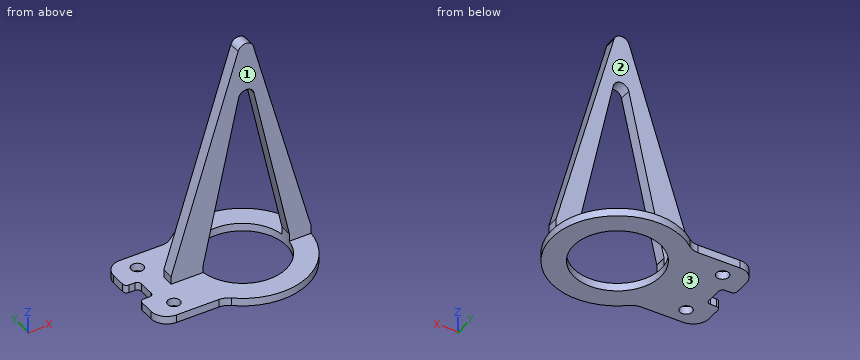
```python
from build123d import *

# Parameters (mm, degrees)
SKETCH_1_R          = 1.56
SKETCH_1_R_2        = 10.981035736
EXTRUDE_1_DEPTH     = 2
EXTRUDE_3_DEPTH     = 2
EXTRUDE_4_DEPTH     = 3
SKETCH_4_W          = 3.5
SKETCH_4_H          = 6
CUT_EXTRUDE_1_DEPTH = 10
FILLET_1_R          = 1
FILLET_2_R          = 1


with BuildPart() as part:
    # 草图1 → 凸台-拉伸1 (new body)
    with BuildSketch(Plane.XY):
        with BuildLine():
            Line((-13.173260362, 11.66726189), (-23.87331228, 11.66726189))
            ThreePointArc((-23.87331228, 11.66726189), (-26.701739405, 10.495689014), (-27.87331228, 7.66726189))
            Line((-27.87331228, 7.66726189), (-27.87331228, -7.66726189))
            ThreePointArc((-27.87331228, -7.66726189), (-26.701739405, -10.495689014), (-23.87331228, -11.66726189))
            Line((-23.87331228, -11.66726189), (-13.173260362, -11.66726189))
            ThreePointArc((-13.173260362, -11.66726189), (-11.803290326, -11.909179653), (-10.599030333, -12.605670839))
            ThreePointArc((-10.599030333, -12.605670839), (16.469437796, 0), (-10.599030333, 12.605670839))
            ThreePointArc((-10.599030333, 12.605670839), (-11.803290326, 11.909179653), (-13.173260362, 11.66726189))
        make_face()
        with Locations((-22, 7.5)):
            Circle(SKETCH_1_R, mode=Mode.SUBTRACT)
        with Locations((-22, -7.5)):
            Circle(SKETCH_1_R, mode=Mode.SUBTRACT)
        Circle(SKETCH_1_R_2, mode=Mode.SUBTRACT)
    extrude(amount=EXTRUDE_1_DEPTH)

    # 草图2 → 凸台-拉伸3 (add)
    with BuildSketch(Plane.XY.offset(2)):
        with BuildLine():
            Line((-19, 1.5), (-10.878103964, 1.5))
            ThreePointArc((-10.878103964, 1.5), (-10.981035736, 0), (-10.878103964, -1.5))
            Line((-10.878103964, -1.5), (-19, -1.5))
            Line((-19, -1.5), (-19, 1.5))
        make_face()
        with BuildLine():
            Line((10.878103964, 1.5), (16.400987206, 1.5))
            ThreePointArc((16.400987206, 1.5), (16.469437796, 0), (16.400987206, -1.5))
            Line((16.400987206, -1.5), (10.878103964, -1.5))
            ThreePointArc((10.878103964, -1.5), (10.981035736, 0), (10.878103964, 1.5))
        make_face()
    extrude(amount=EXTRUDE_3_DEPTH)

    # 草图3 → 凸台-拉伸4 (add)
    with BuildSketch(Plane(origin=(0, 1.5, 0), x_dir=(1, 0, 0), z_dir=(0, 1, 0))):
        with BuildLine():
            Line((-10.878103964, -4), (-1.954283423, -45.017352704))
            ThreePointArc((-1.954283423, -45.017352704), (0, -46.592174739), (1.954283423, -45.017352704))
            Line((1.954283423, -45.017352704), (10.878103964, -4))
            Line((10.878103964, -4), (16.400987206, -4))
            Line((16.400987206, -4), (1.78835733, -57.457623102))
            ThreePointArc((1.78835733, -57.457623102), (-0.101022818, -58.929873662), (-2.047549578, -57.534053964))
            Line((-2.047549578, -57.534053964), (-19, -4))
            Line((-19, -4), (-10.878103964, -4))
        make_face()
    extrude(amount=-EXTRUDE_4_DEPTH)

    # 草图4 → 切除-拉伸1 (cut)
    with BuildSketch(Plane(origin=(0, 0, 0), x_dir=(-1, 0, 0), z_dir=(0, 0, -1))):
        with Locations((26.12331228, 0)):
            Rectangle(SKETCH_4_W, SKETCH_4_H)
    extrude(amount=-CUT_EXTRUDE_1_DEPTH, mode=Mode.SUBTRACT)

    # 圆角1
    fillet_1_edges = [part.edges().sort_by_distance(p)[0] for p in [
        (-27.87331228, 3, 1),
    ]]
    fillet(fillet_1_edges, radius=FILLET_1_R)

    # 圆角2
    fillet_2_edges = [part.edges().sort_by_distance(p)[0] for p in [
        (-24.37331228, 3, 1),
        (-24.37331228, -3, 1),
        (-27.87331228, -3, 1),
    ]]
    fillet(fillet_2_edges, radius=FILLET_2_R)


solid = part.part
```
Work out the finished part from the listing and answer in its coordinate system (mm). Face numbers are marked on the shaded views. A direction names the side the tool comes from. Round coordinates to 2 decimals unless told otherwise and drop trailing zeros. Loops run counter-clockwise (first coordinate to the right, second up) from the corner with the lowest first, then second, coordinate; pieces in that order, holes last. Notation, with made-up numbers: (23.5, 76) -> (33.5, 76) arc R22 cw to (33.5, 113) -> close; hole circle Ø8 at (-31, 73). An arc over 180 degrees is marked (long way). Write each question's results on one line, items separated by ' | '. Start each with the question number.
1. Given pin 1 Ø3 at (x, y) = (-4.5, -11) entering from +Z; pin 2 Ø2 at (y, z) = (0, 2.5) entering from -X; pin 3 Ø3 at (x, z) = (-3, 42.5) entering from +Y, each flat-ended and moving along its own axis, determine where each tip first touches the part or whether it passes through.
2. Find the intervals of material crossed by probe 1 along Y at (x, z) = (-22, 1); probe 2 along Z at (x, y) = (9.5, 8.5); probe 3 along Y at (x, z) = (11.5, 9), in increasing order. Write a range as from..to.
3. Section D-D (x = -17.5) is taken. Determine the outline of the cut face in (y, z).
4. A tool of negligible diameter and unlimited length cuts with its end or side. For the marked faces 1, 2 and 3, from which of +Z, -Z, +X, -X, +Y, -Y can it reach the whole face along a straight path? Write none if from no direction.
5. Section A-A (y = -5) is taken. Determine the outline of the cut face in (x, z).
6. Section C-C (x = 7.5) is taken. Determine the outline of the cut face in (y, z), plus the area to 3 significant figures.
7. Section B-B (z = 21.5) is taken. Determine the outline of the cut face in (x, y), plus the area to 3 significant figures.
Evaluation:
1) pin 1: stops at z = 2 | pin 2: stops at x = -24.37 | pin 3: stops at y = 1.5
2) probe 1: y = -11.67..-9.06, -5.94..5.94, 9.06..11.67 | probe 2: z = 0..2 | probe 3: y = -1.5..1.5
3) outline: (-11.67, 0) -> (11.67, 0) -> (11.67, 2) -> (1.5, 2) -> (1.5, 8.74) -> (-1.5, 8.74) -> (-1.5, 2) -> (-11.67, 2) -> close
4) face 1: +Z, +X, -X, -Y | face 2: +Z, +X, -X, +Y | face 3: -Z, +X, -X, +Y, -Y
5) outline: (-27.87, 0) -> (-9.78, 0) -> (-9.78, 2) -> (-27.87, 2) -> close; (9.78, 0) -> (15.69, 0) -> (15.69, 2) -> (9.78, 2) -> close
6) outline: (-14.66, 0) -> (-8.02, 0) -> (-8.02, 2) -> (-14.66, 2) -> close; (-1.5, 19.53) -> (1.5, 19.53) -> (1.5, 36.56) -> (-1.5, 36.56) -> close; (8.02, 0) -> (14.66, 0) -> (14.66, 2) -> (8.02, 2) -> close | area: 77.7 mm2
7) outline: (-13.46, -1.5) -> (-7.07, -1.5) -> (-7.07, 1.5) -> (-13.46, 1.5) -> close; (7.07, -1.5) -> (11.62, -1.5) -> (11.62, 1.5) -> (7.07, 1.5) -> close | area: 32.8 mm2
